Autodesk Inventor part; units mm, degrees
ref_plane "YZ Plane" through (0, 0, 0) normal (1, 0, 0) x (0, 1, 0)
ref_plane "XZ Plane" through (0, 0, 0) normal (0, 1, 0) x (-1, 0, 0)
ref_plane "XY Plane" through (0, 0, 0) normal (0, 0, 1) x (1, 0, 0)
sketch "Esquisse1" plane through (0, 0, 0) normal (0, 1, 0) x (-1, 0, 0)
  line L0 (1.5706, 55.8) -> (-1.4294, 55.8)
  line L1 (-1.4294, 55.8) -> (-1.4294, -7.8)
  line L2 (-1.4294, -7.8) -> (1.5706, -7.8)
  line L3 (1.5706, -7.8) -> (1.5706, 55.8)
  point P0 (0, 0)
  dimension "d0" = 3
  dimension "d1" = 63.6
extrude "Extrusion1" add sketch "Esquisse1" along normal blind 40
fillet "Congé1" radius 2 2 edges at (-0.0706, 0, 55.8) (-0.0706, 0, -7.8)
fillet "Congé2" radius 1 10 edges at (1.4294, 0.5858, -7.2142) (1.4294, 21, -7.8) (1.4294, 0.5858, 55.2142) (1.4294, 21, 55.8) (1.4294, 0, 24) (-1.5706, 0.5858, 55.2142) (-1.5706, 21, 55.8) (-1.5706, 0.5858, -7.2142) (-1.5706, 21, -7.8) (-1.5706, 0, 24)
sketch "Esquisse2" plane through (1.4294, 2, -6.8) normal (1, 0, 0) x (0, 0, -1)
  line L0 (-62.6, 38) -> (1, 38)
  line L1 (1, 38) -> (1, -2)
  line L2 (1, -2) -> (-62.6, -2)
  line L3 (-62.6, -2) -> (-62.6, 38)
  line L4 (-30.8, 38) -> (-30.8, -2)
  line L5 (-62.6, 18) -> (1, 18)
  circle A0 centre (-35.8, 23) radius 1.75
  circle A1 centre (-45.8, 23) radius 1.75
  circle A2 centre (-55.8, 23) radius 1.75
  circle A3 centre (-55.8, 33) radius 1.75
  circle A4 centre (-45.8, 33) radius 1.75
  circle A5 centre (-35.8, 13) radius 1.75
  circle A6 centre (-45.8, 13) radius 1.75
  circle A7 centre (-55.8, 13) radius 1.75
  circle A8 centre (-55.8, 3) radius 1.75
  circle A9 centre (-45.8, 3) radius 1.75
  circle A10 centre (-35.8, 3) radius 1.75
  circle A11 centre (-25.8, 23) radius 1.75
  circle A12 centre (-15.8, 23) radius 1.75
  circle A13 centre (-5.8, 23) radius 1.75
  circle A14 centre (-5.8, 33) radius 1.75
  circle A15 centre (-15.8, 33) radius 1.75
  circle A16 centre (-25.8, 13) radius 1.75
  circle A17 centre (-25.8, 3) radius 1.75
  circle A18 centre (-15.8, 13) radius 1.75
  circle A19 centre (-15.8, 3) radius 1.75
  circle A20 centre (-5.8, 3) radius 1.75
  circle A21 centre (-5.8, 13) radius 1.75
  line L6 (-40.8, 38) -> (-40.8, 28)
  line L7 (-40.8, 28) -> (-20.8, 28)
  line L8 (-20.8, 28) -> (-20.8, 38)
  line L9 (-20.8, 38) -> (-40.8, 38)
  point P0 (-6.8, -2)
  point P1 (-20.8, 38)
  point P2 (-40.8, 38)
  dimension "d6" = 3.5
  dimension "d7" = 3.5
  dimension "d8" = 3.5
  dimension "d10" = 5
  dimension "d11" = 10
  dimension "d12" = 10
  dimension "d14" = 3.5
  dimension "d15" = 10
  dimension "d16" = 3.5
  dimension "d17" = 10
  dimension "d21" = 5
  dimension "d24" = 10
  dimension "d26" = 20
  dimension "d27" = 10
  dimension "d31" = 40
  dimension "d32" = 63.6
  dimension "d33" = 10
extrude "Extrusion2" cut sketch "Esquisse2" against normal blind 40 contours L0 L4 L7 L6 | L0 L8 L7 L4 | A0 | A1 | A2 | A3 | A4 | A5 | A6 | A7 | A8 | A9 | A10 | A11 | A12 | A13 | A14 | A15 | A16 | A17 | A18 | A19 | A20 | A21
fillet "Congé3" radius 5 4 edges at (-0.0706, 30, 14) (-0.0706, 30, 34) (-0.0706, 40, 14) (-0.0706, 40, 34)
properties part number "plaque_Impression 3D"
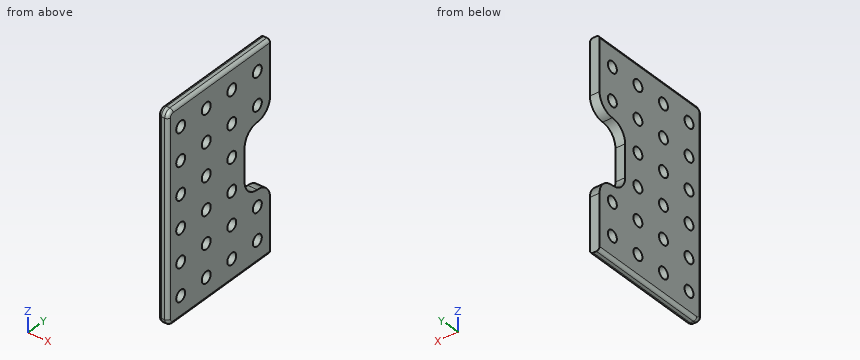
Could you check a few things on this model? Use its own coordinates, in mm. Give positions to 0.01 mm unless a question says otherwise; leave off trailing zeros. Loops run counter-clockwise (first coordinate to the right, second up) from the corner with the lowest first, then second, coordinate; pieces in that order, holes last. Notation, with made-up numbers: (-3, -17) -> (8, -17) arc R24 cw to (8, 11) -> close; hole circle Ø3 at (17, 64). An arc over 180 degrees is marked (long way). Return JSON: item names as keys, results as strings.
Item 1: If we section it at A-A on z = 49: List the corners of the cut face in (x, y) for me, plus the area to 3 significant figures.
Geometry results:
{"outline": "(-1.57, 1) arc R1 ccw to (-0.57, 0) -> (0.43, 0) arc R1 ccw to (1.43, 1) -> (1.43, 3.25) -> (-1.57, 3.25) -> close; (-1.57, 6.75) -> (1.43, 6.75) -> (1.43, 13.25) -> (-1.57, 13.25) -> close; (-1.57, 16.75) -> (1.43, 16.75) -> (1.43, 23.25) -> (-1.57, 23.25) -> close; (-1.57, 26.75) -> (1.43, 26.75) -> (1.43, 33.25) -> (-1.57, 33.25) -> close; (-1.57, 36.75) -> (1.43, 36.75) -> (1.43, 40) -> (-1.57, 40) -> close", "area": "77.6 mm²"}
Item 2: If we section it at B-B on y = 5: Count the separate pieces of the cut face and the enclosed holes in it, plus the area to 3 significant figures.
Geometry results:
{"separate pieces": "7", "enclosed holes": "0", "area": "127 mm²"}
Item 3: I need wall thicknesses on L1, parallel to Y at x = -0.3, z = 9; L2, parallel to Y at x = -0.05, z = 10; L3, parallel to Z at x = -0.7, y = 22. Which ranges of each line are inside material? Lowest first, please. Write a range as from..to.
Geometry results:
{"L1": "y = 0..3.25, 6.75..13.25, 16.75..23.25, 26.75..33.25, 36.75..40", "L2": "y = 0..3.56, 6.44..13.56, 16.44..23.56, 26.44..33.56, 36.44..39.9", "L3": "z = -7.79..55.79"}
